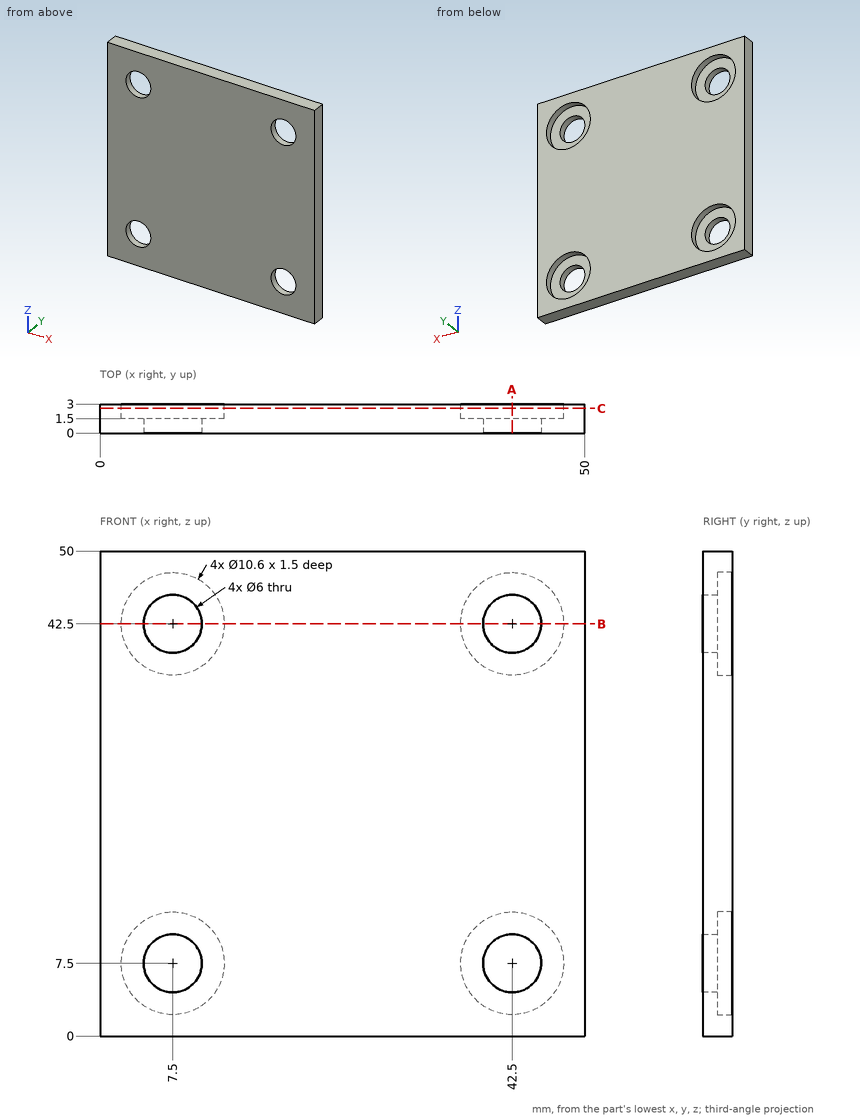
Design review of the part shown in the three views and the two pictorial views. Dimensions are in mm from the part's minimum x, y and z. Round coordinates to 2 decimals unless told otherwise and drop trailing zeros. Loops run counter-clockwise (first coordinate to the right, second up) from the corner with the lowest first, then second, coordinate; pieces in that order, holes last.
Q1. Add section B-B on z = 42.5. Write out the cut boundary in (x, y).
Result sheet:
outline: (0, 0) - (4.5, 0) - (4.5, 1.5) - (2.2, 1.5) - (2.2, 3) - (0, 3) - close; (10.5, 0) - (39.5, 0) - (39.5, 1.5) - (37.2, 1.5) - (37.2, 3) - (12.8, 3) - (12.8, 1.5) - (10.5, 1.5) - close; (45.5, 0) - (50, 0) - (50, 3) - (47.8, 3) - (47.8, 1.5) - (45.5, 1.5) - close
Q2. Add section C-C on y = 2.55. Write out the cut boundary in (x, z), plus the area to 3 significant figures.
Result sheet:
outline: (0, 0) - (50, 0) - (50, 50) - (0, 50) - close; hole circle Ø10.6 at (7.5, 7.5); hole circle Ø10.6 at (7.5, 42.5); hole circle Ø10.6 at (42.5, 7.5); hole circle Ø10.6 at (42.5, 42.5)
area: 2,150 mm2
Q3. Add section A-A on x = 42.5. Write out the cut boundary in (y, z).
Result sheet:
outline: (0, 0) - (3, 0) - (3, 2.2) - (1.5, 2.2) - (1.5, 4.5) - (0, 4.5) - close; (0, 10.5) - (1.5, 10.5) - (1.5, 12.8) - (3, 12.8) - (3, 37.2) - (1.5, 37.2) - (1.5, 39.5) - (0, 39.5) - close; (0, 45.5) - (1.5, 45.5) - (1.5, 47.8) - (3, 47.8) - (3, 50) - (0, 50) - close
Q4. To check wall thickness, follow line 1 along Z through (x, y) = (42.5, 0.75); line 2 along X through (y, z) = (2.6, 7.5). State the ranges of each line that lie inside material, in increasing order.
Result sheet:
line 1: z = 0 to 4.5, 10.5 to 39.5, 45.5 to 50
line 2: x = 0 to 2.2, 12.8 to 37.2, 47.8 to 50
Q5. Insertion check: pin 1 Ø1 at (y, z) = (1.5, 43.5) entering from -X; pin 2 Ø8.5 at (x, z) = (7.5, 7.5) entering from +Y. Each pin has a flat end and moves straight along its axis. Give the tip position at first contact, or say it passes through.
Result sheet:
pin 1: stops at x = 0
pin 2: stops at y = 1.5
